Geometry: final body of the model. Coordinates: model frame, mm. A direction names the side the tool comes from. Coordinates: 2 decimals unless noted, no trailing zeros. Order: outer loops, then holes, each group sorted by start corner. A loop starts at its lowest first (then second) coordinate and runs counter-clockwise, first axis right, second up. Notation, with made-up numbers: M 82.25,37.5 L 109.25,37.5 A29 ccw 109.25,74.5 Z; hole C -20,88 d5. An arc over 180 degrees is marked long. Write item = value, one per line.
from build123d import *

# Parameters (mm, degrees)
F0_W      = 40
F0_H      = 28
F1_DEPTH  = 6
F3_DEPTH  = 38
F4_R      = 1.5
F5_DEPTH  = 2
F7_R      = 2.225
F7_R_2    = 1.225
F8_DEPTH  = 3
F9_R      = 2
F10_DEPTH = 17
F11_R     = 1.5
F12_DEPTH = 1.5
F13_DEPTH = 6.7
F15_DEPTH = 8
F16_R     = 3
F17_DEPTH = 4.5
F19_DEPTH = 15
F20_R     = 1.3333333333


with BuildPart() as f1:
    # F0 (on Front) → F1 (new body)
    with BuildSketch(Plane.XZ):
        with Locations((20, -14)):
            Rectangle(F0_W, F0_H)
    extrude(amount=F1_DEPTH)

    # F2 (on face) → F3 (cut, through all)
    with BuildSketch(Plane.YZ.offset(40)):
        with BuildLine():
            Line((-6, -23), (-6, -28))
            Line((-6, -28), (-1, -28))
            Line((-1, -28), (-1, -25.5))
            ThreePointArc((-1, -25.5), (-1.732233047, -23.732233047), (-3.5, -23))
            Line((-3.5, -23), (-6, -23))
        make_face()
        with BuildLine():
            Line((-6, 0), (-6, -5))
            Line((-6, -5), (-3.5, -5))
            ThreePointArc((-3.5, -5), (-1.732233047, -4.267766953), (-1, -2.5))
            Line((-1, -2.5), (-1, 0))
            Line((-1, 0), (-6, 0))
        make_face()
    extrude(amount=-F3_DEPTH, mode=Mode.SUBTRACT)

    # F4 (on face) → F5 (cut)
    with BuildSketch(Plane(origin=(0, 0, 0), x_dir=(0, -1, 0), z_dir=(-1, 0, 0))):
        with Locations((3.5, -25.5)):
            Circle(F4_R)
        with BuildLine():
            ThreePointArc((0, -22.94427191), (4, -14), (0, -5.05572809))
            Line((0, -5.05572809), (0, -22.94427191))
        make_face()
        with Locations((3.5, -2.5)):
            Circle(F4_R)
    extrude(amount=-F5_DEPTH, mode=Mode.SUBTRACT)

    # F7 (on face) → F8 (join)
    with BuildSketch(Plane(origin=(0, 0, 0), x_dir=(-1, 0, 0), z_dir=(0, 1, 0))):
        with Locations((-20.5, -24)):
            Circle(F7_R)
        with Locations((-20.5, -24)):
            Circle(F7_R_2, mode=Mode.SUBTRACT)
        with Locations((-30.4902837155, -23.5592832158)):
            Circle(F7_R)
        with Locations((-30.4902837155, -23.5592832158)):
            Circle(F7_R_2, mode=Mode.SUBTRACT)
    extrude(amount=F8_DEPTH)

    # F9 (on face) → F10 (join)
    with BuildSketch(Plane(origin=(0, 0, 0), x_dir=(-1, 0, 0), z_dir=(0, 1, 0))):
        with Locations((-38, -26)):
            Circle(F9_R)
        with Locations((-9, -24)):
            Circle(F9_R)
        with Locations((-9, -4)):
            Circle(F9_R)
    extrude(amount=F10_DEPTH)

    # F11 (on face) → F12 (join)
    with BuildSketch(Plane(origin=(0, 17, 0), x_dir=(-1, 0, 0), z_dir=(0, 1, 0))):
        with Locations((-38, -26)):
            Circle(F11_R)
        with Locations((-9, -24)):
            Circle(F11_R)
        with Locations((-9, -4)):
            Circle(F11_R)
    extrude(amount=F12_DEPTH)

    # F13 (add): a face of the model
    f13_faces = [f1.faces().sort_by_distance(p)[0] for p in [
        (0, -0.2863564213, -2.527864045),
    ]]
    extrude(f13_faces, amount=F13_DEPTH)

    # F14 (on face) → F15 (join)
    with BuildSketch(Plane.YZ.offset(40)):
        with BuildLine():
            Line((0, 0), (-1, 0))
            Line((-1, 0), (-1, -2.5))
            ThreePointArc((-1, -2.5), (-1.732233047, -4.267766953), (-3.5, -5))
            Line((-3.5, -5), (-6, -5))
            Line((-6, -5), (-6, -23))
            Line((-6, -23), (-3.5, -23))
            ThreePointArc((-3.5, -23), (-1.732233047, -23.732233047), (-1, -25.5))
            Line((-1, -25.5), (-1, -28))
            Line((-1, -28), (0, -28))
            Line((0, -28), (0, 0))
        make_face()
    extrude(amount=F15_DEPTH)

    # F16 (on face) → F17 (cut)
    with BuildSketch(Plane(origin=(0, 0, 0), x_dir=(-1, 0, 0), z_dir=(0, 1, 0))):
        with Locations((-38, -10)):
            Circle(F16_R)
    extrude(amount=-F17_DEPTH, mode=Mode.SUBTRACT)

    # F18 (on face) → F19 (join)
    with BuildSketch(Plane.YZ.offset(48)):
        with BuildLine():
            Line((-3.5, -23), (-6, -23))
            Line((-6, -23), (-6, -29.8))
            Line((-6, -29.8), (0, -29.8))
            Line((0, -29.8), (0, -28))
            Line((0, -28), (-1, -28))
            Line((-1, -28), (-1, -25.5))
            ThreePointArc((-1, -25.5), (-1.732233047, -23.732233047), (-3.5, -23))
        make_face()
    extrude(amount=-F19_DEPTH)

    # F20
    f20_edges = [f1.edges().sort_by_distance(p)[0] for p in [
        (40, 0, -26),
        (11, 0, -24),
        (11, 0, -4),
    ]]
    fillet(f20_edges, radius=F20_R)


solid = f1.part
1) Pin query (flat end, axial travel): pin 1 (4 mm diameter, centred on y = 11, z = -4.5, fed in from -X); pin 2 (0.8 mm diameter, centred on x = 19, y = -5, fed in from -Z); pin 3 (5 mm diameter, centred on x = 35, y = 7.5, fed in from +Z); pin 4 (5 mm diameter, centred on x = -0.5, y = 4, fed in from -Z). Return the tip coordinate at first contact, or that it passes through.
Numbers:
pin_1 = 7
pin_2 = -23
pin_3 = -24.06
pin_4 = through
2) Set-up query: faces 1 (the face through (2, -5, -27)), 2 (the face through (38, -4.5, -10)), 3 (the face through (2, -2, -14)). Return all of +Z, -Z, +X, -X, +Y, -Y with unobstructed straight access to the full face (end or side cutting, diameter ignored); none if empty.
Numbers:
face_1 = -Z, -Y
face_2 = +Y
face_3 = -X, +Y
3) Section C-C, the plane x = 14. Return loops of the section in (y, z), and give its area (3 significant figures).
Numbers:
outline = M -6,-23 L -3.5,-23 A2.5 cw -1,-25.5 L -1,-28 L 0,-28 L 0,0 L -1,0 L -1,-2.5 A2.5 cw -3.5,-5 L -6,-5 Z
area = 121 mm²
4) Mould query, pull axis Z, two halves, no side actions, for faces 4 (the face through (10.5, 17.74, -3.93)), 5 (the face through (17.283, -1.752, -23.713)), 6 (the face through (25, -5, -5)). Classes: pulls with the +Z half, pulls with the -Z half, needs draft (parallel to the pull), parting line crosses it, or undercut.
Numbers:
face_4 = undercut
face_5 = pulls with the -Z half
face_6 = pulls with the +Z half
5) Section B-B, the plane y = 9. Return loops of the section in (x, z), and give its area (3 significant figures).
Numbers:
outline = C 9,-24 d4; C 9,-4 d4; C 38,-26 d4
area = 37.7 mm²
6) Section A-A, the plane x = 20.5. Return loops of the section in (y, z) (3 decimals), and give its area (3 significant figures).
Numbers:
outline = M -6,-23 L -3.5,-23 A2.5 cw -1,-25.5 L -1,-28 L 0,-28 L 0,-26.225 L 3,-26.225 L 3,-25.225 L 0,-25.225 L 0,-22.775 L 3,-22.775 L 3,-21.775 L 0,-21.775 L 0,0 L -1,0 L -1,-2.5 A2.5 cw -3.5,-5 L -6,-5 Z
area = 127 mm²
7) Line query: L1, parallel to Y at x = 16, z = -27; L2, parallel to Y at x = 41, z = -19; L3, parallel to X at y = 3.5, z = -25. Output: solid intervals per line, ascending.
Numbers:
L1 = -1 to 0
L2 = -6 to 0
L3 = 7.27 to 10.73, 36.27 to 39.73
